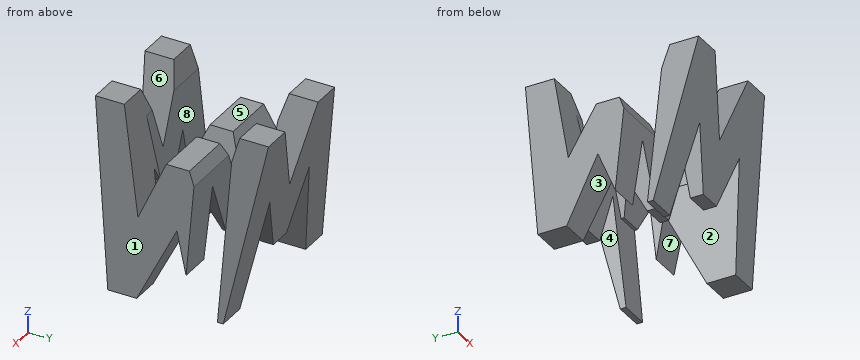
from build123d import *

# Parameters (mm, degrees)
F0_W      = 38.1
F0_H      = 38.1
F1_DEPTH  = 38.1
F6_DEPTH  = 38.1
F8_DEPTH  = 38.1
F9_W      = 25.4
F9_H      = 7.62
F10_DEPTH = 38.1


with BuildPart() as f1:
    # F0 (on Front) → F1 (new body)
    with BuildSketch(Plane.XZ):
        with Locations((19.05, 19.05)):
            Rectangle(F0_W, F0_H)
    extrude(amount=F1_DEPTH)

    # F5 (on offset) → F6 (cut)
    with BuildSketch(Plane.YZ.offset(38.1)):
        Polygon((-11.43, 17.112495), (-6.35, 38.1), (-31.75, 38.1), (-26.67, 16.286777), (-21.59, 28.575), (-16.51, 28.575), align=None)
        Polygon((-31.75, 0), (-38.1, 38.1), (-38.1, 0), align=None)
        Polygon((-25.4, 0), (-12.7, 0), (-18.055946, 15.875), align=None)
        Polygon((-6.35, 0), (0, 0), (0, 38.1), align=None)
    extrude(amount=-F6_DEPTH, mode=Mode.SUBTRACT)

    # F7 (on offset) → F8 (cut)
    with BuildSketch(Plane.XZ.offset(38.1)):
        Polygon((11.43, 22.225), (6.35, 0), (31.75, 0), (26.67, 22.225), (21.59, 9.525), (16.51, 9.525), align=None)
        Polygon((0, 38.1), (0, 0), (6.35, 38.1), align=None)
        Polygon((25.4, 38.1), (12.7, 38.1), (19.05, 22.225), align=None)
        Polygon((31.75, 38.1), (38.1, 0), (38.1, 38.1), align=None)
    extrude(amount=-F8_DEPTH, mode=Mode.SUBTRACT)

    # F9 (on offset) → F10 (cut)
    with BuildSketch(Plane.XY.offset(38.1)):
        with Locations((25.4, -11.43)):
            Rectangle(F9_W, F9_H)
        with Locations((12.7, -26.67)):
            Rectangle(F9_W, F9_H)
    extrude(amount=-F10_DEPTH, mode=Mode.SUBTRACT)


solid = f1.part
CAD build for the part. Positions are in the model's coordinates, mm. Face numbers are marked on the shaded views. A direction names the side the tool comes from. Round coordinates to 2 decimals unless told otherwise and drop trailing zeros. Loops run counter-clockwise (first coordinate to the right, second up) from the corner with the lowest first, then second, coordinate; pieces in that order, holes last.
(1) Cut at C-C (y = -3.5). Give the cut face in (x, z) (3 decimals), plus the area to 3 significant figures.
(2) Drop flat-ended pins along their axis: pin 1 (1.5 mm diameter, centred on x = 8, y = -18.5, fed in from +Z) (3 decimals); pin 2 (5 mm diameter, centred on y = -13.5, z = 12.5, fed in from -X); pin 3 (1.5 mm diameter, centred on x = 26.5, z = 25, fed in from +Y). Give the stop position or say it passes through.
(3) Cut at A-A (x = 29). Give the cut face in (y, z) (3 decimals).
(4) Wall check: line 1 along Y through (x, z) = (17.5, 26); line 2 along Y through (x, z) = (10.5, 20); line 3 along X through (y, z) = (-7, 14). Give the ranges that are in metal, low to high.
(5) Two-plate mould, pull along X, no slides. Class the marked faces 1, 2 and 3: +X half, -X half, draft (parallel to the pull), parting line (faces both ways), or undercut.
(6) Cut at B-B (z = 7). Give the cut face in (x, y), plus the area to 3 significant figures.
(7) Cut at D-D (z = 26.5). Give the cut face in (x, y).
(8) Which spindle directions (+Z, -Z, +X, -X, +Y, -Y) get a long thin tool onto all of the face, cutting with end or side? Do the marked faces 4, 5, 6, 7 and 8. Say none if no direction does.
Findings below:
1. outline: (2.85, 17.1) - (10.259, 17.1) - (11.43, 22.225) - (13.48, 17.1) - (24.62, 17.1) - (26.67, 22.225) - (27.841, 17.1) - (35.25, 17.1) - (31.75, 38.1) - (25.4, 38.1) - (19.05, 22.225) - (12.7, 38.1) - (6.35, 38.1) - close
1. area: 490 mm2
2. pin 1: stops at z = 28.575
2. pin 2: stops at x = 1.67
2. pin 3: stops at y = -2.06
3. outline: (-38.1, 38.1) - (-33.755, 12.031) - (-19.834, 12.031) - (-18.056, 15.875) - (-16.759, 12.031) - (-15.24, 12.031) - (-15.24, 25.709) - (-16.51, 28.575) - (-21.59, 28.575) - (-26.67, 16.287) - (-31.75, 38.1) - close; (-7.62, 12.031) - (-4.345, 12.031) - (0, 38.1) - (-6.35, 38.1) - (-7.62, 32.853) - close
4. line 1: y = -36.08 to -30.48, -22.65 to -15.37, -7.62 to -2.02
4. line 2: y = -35.08 to -30.48, -22.86 to -12.71, -10.73 to -3.02
4. line 3: x = 2.33 to 9.55, 14.72 to 23.38, 28.55 to 35.77
5. face 1: +X half
5. face 2: undercut
5. face 3: draft
6. outline: (1.17, -32.92) - (7.95, -32.92) - (7.95, -30.48) - (1.17, -30.48) - close; (1.17, -22.86) - (7.95, -22.86) - (7.95, -22.16) - (1.17, -22.16) - close; (1.17, -15.06) - (7.95, -15.06) - (7.95, -5.18) - (1.17, -5.18) - close; (30.15, -32.92) - (36.93, -32.92) - (36.93, -22.16) - (30.15, -22.16) - close; (30.15, -7.62) - (36.93, -7.62) - (36.93, -5.18) - (30.15, -5.18) - close
6. area: 178 mm2
7. outline: (4.42, -36.17) - (17.34, -36.17) - (17.34, -30.48) - (4.42, -30.48) - close; (4.42, -22.45) - (17.34, -22.45) - (17.34, -15.59) - (4.42, -15.59) - close; (4.42, -9.16) - (12.7, -9.16) - (12.7, -7.62) - (17.34, -7.62) - (17.34, -1.93) - (4.42, -1.93) - close; (20.76, -36.17) - (33.68, -36.17) - (33.68, -29.05) - (25.4, -29.05) - (25.4, -30.48) - (20.76, -30.48) - close; (20.76, -22.45) - (33.68, -22.45) - (33.68, -15.59) - (20.76, -15.59) - close; (20.76, -7.62) - (33.68, -7.62) - (33.68, -1.93) - (20.76, -1.93) - close
8. face 4: -Z, +Y, -Y
8. face 5: +Z, +X, -X
8. face 6: +Z, +Y, -Y
8. face 7: -Z, +X, -X
8. face 8: +Z, -Z, -X
